The drawing under review shows one solid part. Ordinate dimensions are in mm from its lowest x, y, z. A direction names the side the tool comes from. Coordinates: 2 decimals unless noted, no trailing zeros. Write each loop counter-clockwise with the first axis right and the second up, starting at its lowest first coordinate (ties: lowest second). Pieces come first, ordered by that corner, then holes.
Q1. Insertion check: pin 1 (6.5 mm diameter, centred on x = 12.7, y = 12.7, fed in from +Z). The pin has a flat end and moves straight along its axis. Give the tip position at first contact, or say it passes through.
Q2. For probe 1 along X at (y, z) = (12.75, 22.75); probe 2 along Y at (x, z) = (21, 22) (1 decimal), list the stretches that pass through material, from the lowest coordinate up.
Q3. Take a section at C-C (y = 21.5). Give the boundary of the cut face in (x, z) (1 decimal).
Q4. Take a section at A-A (z = 12.7). State how many separate pieces and enclosed holes the cut face has.
Q5. Mouldability with a two-part tool opening along Z and no side actions: class the marked faces 1, 2 and 3 as pulls with the +Z half, pulls with the -Z half, needs draft (parallel to the pull), parting line crosses it, or undercut.
Q6. Machinability: for the marked faces 4 and 5, which of the approach directions +Z, -Z, +X, -X, +Y, -Y give a long, thin tool a straight path to every point of the face, cutting with its end or side? Answer none if there is none.
Q7. Take a section at B-B (x = 12.7). Give the boundary of the cut face in (y, z) (1 decimal).
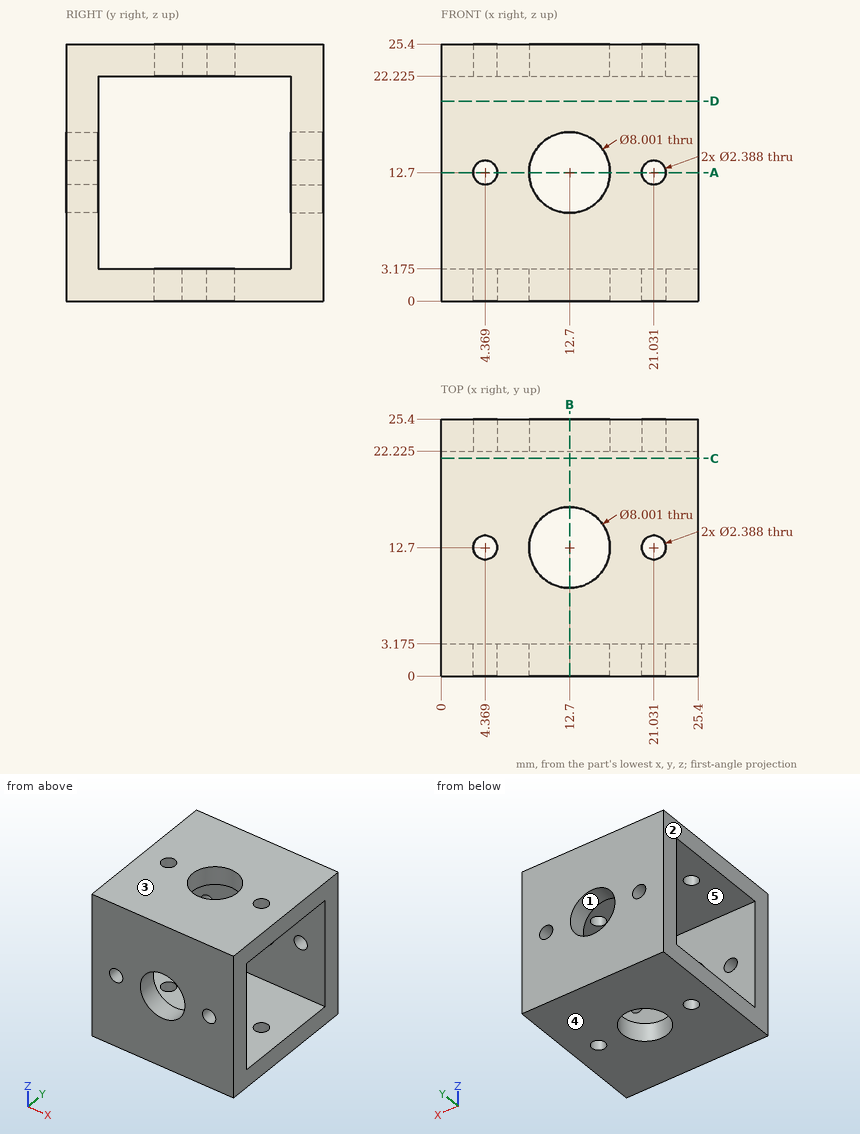
Response:
1. pin 1: passes through
2. probe 1: x = 0 to 3.18, 5.56 to 8.7, 16.7 to 19.84, 22.22 to 25.4
2. probe 2: y = 0 to 3.2, 22.2 to 25.4
3. outline: (0, 0) - (25.4, 0) - (25.4, 3.2) - (0, 3.2) - close; (0, 22.2) - (25.4, 22.2) - (25.4, 25.4) - (0, 25.4) - close
4. separate pieces: 8
4. enclosed holes: 0
5. face 1: undercut
5. face 2: needs draft
5. face 3: pulls with the +Z half
6. face 4: -Z, +X, -X, +Y, -Y
6. face 5: +X, -X
7. outline: (0, 0) - (8.7, 0) - (8.7, 3.2) - (3.2, 3.2) - (3.2, 8.7) - (0, 8.7) - close; (0, 16.7) - (3.2, 16.7) - (3.2, 22.2) - (8.7, 22.2) - (8.7, 25.4) - (0, 25.4) - close; (16.7, 0) - (25.4, 0) - (25.4, 8.7) - (22.2, 8.7) - (22.2, 3.2) - (16.7, 3.2) - close; (16.7, 22.2) - (22.2, 22.2) - (22.2, 16.7) - (25.4, 16.7) - (25.4, 25.4) - (16.7, 25.4) - close
